Part model, mm, in its own coordinate system. A direction names the side the tool comes from. Give positions to 0.01 mm unless a question says otherwise; leave off trailing zeros. Order: outer loops, then holes, each group sorted by start corner. A loop starts at its lowest first (then second) coordinate and runs counter-clockwise, first axis right, second up. Notation, with made-up numbers: M 73.5,68 L 131.5,68 A19 ccw 131.5,75 Z; hole C 35,15.25 d2. An arc over 180 degrees is marked long. One line per question, with ' | ' between items.
```python
from build123d import *

# Parameters (mm, degrees)
SKETCH1_W               = 2200
SKETCH1_H               = 1000
BOSS_EXTRUDE1_DEPTH     = 1100
SKETCH2_W               = 2000
SKETCH2_H               = 900
CUT_EXTRUDE1_DEPTH      = 1
CUT_EXTRUDE1_DEPTH_BACK = 1101
FILLET1_R               = 50
CUT_EXTRUDE2_REACH      = 1002
SKETCH3_W               = 100
SKETCH3_H               = 900
SKETCH4_W               = 1000
SKETCH4_H               = 850
CUT_EXTRUDE3_DEPTH      = 1
CUT_EXTRUDE3_DEPTH_BACK = 2201


with BuildPart() as part:
    # Sketch1 → Boss-Extrude1 (new body)
    with BuildSketch(Plane.XY):
        with Locations((-1100, 500)):
            Rectangle(SKETCH1_W, SKETCH1_H)
    extrude(amount=BOSS_EXTRUDE1_DEPTH)

    # Sketch2 → Cut-Extrude1 (cut, two sides)
    with BuildSketch(Plane.XY.offset(1100)) as cut_extrude1_sk:
        with Locations((-1100, 500)):
            Rectangle(SKETCH2_W, SKETCH2_H)
    extrude(amount=CUT_EXTRUDE1_DEPTH, mode=Mode.SUBTRACT)
    extrude(cut_extrude1_sk.sketch, amount=-CUT_EXTRUDE1_DEPTH_BACK, mode=Mode.SUBTRACT)

    # Fillet1
    fillet1_edges = [part.edges().sort_by_distance(p)[0] for p in [
        (-2100, 50, 550),
        (-2100, 950, 550),
        (-100, 950, 550),
        (-100, 50, 550),
        (0, 0, 550),
        (-2200, 0, 550),
        (-2200, 1000, 550),
        (0, 1000, 550),
    ]]
    fillet(fillet1_edges, radius=FILLET1_R)

    # Sketch3 → Cut-Extrude2 (cut, up to next)
    with BuildSketch(Plane(origin=(0, 1000, 0), x_dir=(1, 0, 0), z_dir=(0, 1, 0)), mode=Mode.PRIVATE) as cut_extrude2_sk1:
        with Locations((-2000, -550)):
            Rectangle(SKETCH3_W, SKETCH3_H)
    cut_extrude2_tool1 = extrude(cut_extrude2_sk1.sketch, amount=-CUT_EXTRUDE2_REACH, mode=Mode.PRIVATE) & part.part
    add(cut_extrude2_tool1.solids().sort_by_distance((-2000, 1000, 550))[0], mode=Mode.SUBTRACT)
    # Sketch3 → Cut-Extrude2 (cut, up to next)
    with BuildSketch(Plane(origin=(0, 1000, 0), x_dir=(1, 0, 0), z_dir=(0, 1, 0)), mode=Mode.PRIVATE) as cut_extrude2_sk2:
        with Locations((-1800, -550)):
            Rectangle(SKETCH3_W, SKETCH3_H)
    cut_extrude2_tool2 = extrude(cut_extrude2_sk2.sketch, amount=-CUT_EXTRUDE2_REACH, mode=Mode.PRIVATE) & part.part
    add(cut_extrude2_tool2.solids().sort_by_distance((-1800, 1000, 550))[0], mode=Mode.SUBTRACT)
    # Sketch3 → Cut-Extrude2 (cut, up to next)
    with BuildSketch(Plane(origin=(0, 1000, 0), x_dir=(1, 0, 0), z_dir=(0, 1, 0)), mode=Mode.PRIVATE) as cut_extrude2_sk3:
        with Locations((-1600, -550)):
            Rectangle(SKETCH3_W, SKETCH3_H)
    cut_extrude2_tool3 = extrude(cut_extrude2_sk3.sketch, amount=-CUT_EXTRUDE2_REACH, mode=Mode.PRIVATE) & part.part
    add(cut_extrude2_tool3.solids().sort_by_distance((-1600, 1000, 550))[0], mode=Mode.SUBTRACT)
    # Sketch3 → Cut-Extrude2 (cut, up to next)
    with BuildSketch(Plane(origin=(0, 1000, 0), x_dir=(1, 0, 0), z_dir=(0, 1, 0)), mode=Mode.PRIVATE) as cut_extrude2_sk4:
        with Locations((-1400, -550)):
            Rectangle(SKETCH3_W, SKETCH3_H)
    cut_extrude2_tool4 = extrude(cut_extrude2_sk4.sketch, amount=-CUT_EXTRUDE2_REACH, mode=Mode.PRIVATE) & part.part
    add(cut_extrude2_tool4.solids().sort_by_distance((-1400, 1000, 550))[0], mode=Mode.SUBTRACT)
    # Sketch3 → Cut-Extrude2 (cut, up to next)
    with BuildSketch(Plane(origin=(0, 1000, 0), x_dir=(1, 0, 0), z_dir=(0, 1, 0)), mode=Mode.PRIVATE) as cut_extrude2_sk5:
        with Locations((-1200, -550)):
            Rectangle(SKETCH3_W, SKETCH3_H)
    cut_extrude2_tool5 = extrude(cut_extrude2_sk5.sketch, amount=-CUT_EXTRUDE2_REACH, mode=Mode.PRIVATE) & part.part
    add(cut_extrude2_tool5.solids().sort_by_distance((-1200, 1000, 550))[0], mode=Mode.SUBTRACT)
    # Sketch3 → Cut-Extrude2 (cut, up to next)
    with BuildSketch(Plane(origin=(0, 1000, 0), x_dir=(1, 0, 0), z_dir=(0, 1, 0)), mode=Mode.PRIVATE) as cut_extrude2_sk6:
        with Locations((-1000, -550)):
            Rectangle(SKETCH3_W, SKETCH3_H)
    cut_extrude2_tool6 = extrude(cut_extrude2_sk6.sketch, amount=-CUT_EXTRUDE2_REACH, mode=Mode.PRIVATE) & part.part
    add(cut_extrude2_tool6.solids().sort_by_distance((-1000, 1000, 550))[0], mode=Mode.SUBTRACT)
    # Sketch3 → Cut-Extrude2 (cut, up to next)
    with BuildSketch(Plane(origin=(0, 1000, 0), x_dir=(1, 0, 0), z_dir=(0, 1, 0)), mode=Mode.PRIVATE) as cut_extrude2_sk7:
        with Locations((-800, -550)):
            Rectangle(SKETCH3_W, SKETCH3_H)
    cut_extrude2_tool7 = extrude(cut_extrude2_sk7.sketch, amount=-CUT_EXTRUDE2_REACH, mode=Mode.PRIVATE) & part.part
    add(cut_extrude2_tool7.solids().sort_by_distance((-800, 1000, 550))[0], mode=Mode.SUBTRACT)
    # Sketch3 → Cut-Extrude2 (cut, up to next)
    with BuildSketch(Plane(origin=(0, 1000, 0), x_dir=(1, 0, 0), z_dir=(0, 1, 0)), mode=Mode.PRIVATE) as cut_extrude2_sk8:
        with Locations((-600, -550)):
            Rectangle(SKETCH3_W, SKETCH3_H)
    cut_extrude2_tool8 = extrude(cut_extrude2_sk8.sketch, amount=-CUT_EXTRUDE2_REACH, mode=Mode.PRIVATE) & part.part
    add(cut_extrude2_tool8.solids().sort_by_distance((-600, 1000, 550))[0], mode=Mode.SUBTRACT)
    # Sketch3 → Cut-Extrude2 (cut, up to next)
    with BuildSketch(Plane(origin=(0, 1000, 0), x_dir=(1, 0, 0), z_dir=(0, 1, 0)), mode=Mode.PRIVATE) as cut_extrude2_sk9:
        with Locations((-400, -550)):
            Rectangle(SKETCH3_W, SKETCH3_H)
    cut_extrude2_tool9 = extrude(cut_extrude2_sk9.sketch, amount=-CUT_EXTRUDE2_REACH, mode=Mode.PRIVATE) & part.part
    add(cut_extrude2_tool9.solids().sort_by_distance((-400, 1000, 550))[0], mode=Mode.SUBTRACT)
    # Sketch3 → Cut-Extrude2 (cut, up to next)
    with BuildSketch(Plane(origin=(0, 1000, 0), x_dir=(1, 0, 0), z_dir=(0, 1, 0)), mode=Mode.PRIVATE) as cut_extrude2_sk10:
        with Locations((-200, -550)):
            Rectangle(SKETCH3_W, SKETCH3_H)
    cut_extrude2_tool10 = extrude(cut_extrude2_sk10.sketch, amount=-CUT_EXTRUDE2_REACH, mode=Mode.PRIVATE) & part.part
    add(cut_extrude2_tool10.solids().sort_by_distance((-200, 1000, 550))[0], mode=Mode.SUBTRACT)

    # Sketch4 → Cut-Extrude3 (cut, two sides)
    with BuildSketch(Plane(origin=(0, 0, 0), x_dir=(0, 0, -1), z_dir=(1, 0, 0))) as cut_extrude3_sk:
        with Locations((-550, 500)):
            Rectangle(SKETCH4_W, SKETCH4_H)
    extrude(amount=CUT_EXTRUDE3_DEPTH, mode=Mode.SUBTRACT)
    extrude(cut_extrude3_sk.sketch, amount=-CUT_EXTRUDE3_DEPTH_BACK, mode=Mode.SUBTRACT)


solid = part.part
```
1. Mould opens along Z. For faces 1 (the flat face through (-2200, 65, 547)), 2 (the flat face through (-1105, 984, 1100)), 3 (the flat face through (-1950, 975, 556)) say: released by +Z, released by -Z, zero draft, split by the parting line, or undercut.
Worked out:
face 1: zero draft | face 2: released by +Z | face 3: undercut
2. Slice it at B-B on y = 560.5. Give the cut face in (x, z).
Worked out:
outline: M -2200,0 L -2100,0 L -2100,50 L -2200,50 Z; M -2200,1050 L -2100,1050 L -2100,1100 L -2200,1100 Z; M -100,0 L 0,0 L 0,50 L -100,50 Z; M -100,1050 L 0,1050 L 0,1100 L -100,1100 Z
3. Slice it at A-A on x = -1377. Give the cut face in (y, z).
Worked out:
outline: M 0,0 L 50,0 L 50,1100 L 0,1100 Z; M 950,0 L 1000,0 L 1000,100 L 950,100 Z; M 950,1000 L 1000,1000 L 1000,1100 L 950,1100 Z
4. Slice it at D-D on z = 947. Give the number of separate pieces and of enclosed holes in the cut face, then the cut area to 3 significant figures.
Worked out:
separate pieces: 12 | enclosed holes: 0 | area: 180,000 mm2
5. Drop flat-ended pins along their axis: pin 1 (1.5 mm diameter, centred on x = -1800, z = 498.5, fed in from +Y); pin 2 (15 mm diameter, centred on y = 975, z = 698, fed in from -X); pin 3 (25 mm diameter, centred on x = -604, y = 968, fed in from -Z); pin 4 (15 mm diameter, centred on y = 971.5, z = 438.5, fed in from +X). Give the stop position or say it passes through.
Worked out:
pin 1: stops at y = 50 | pin 2: stops at x = -2196.84 | pin 3: stops at z = 0 | pin 4: stops at x = -2
6. Slice it at C-C on x = -479. Give the cut face in (y, z).
Worked out:
outline: M 0,0 L 50,0 L 50,1100 L 0,1100 Z; M 950,0 L 1000,0 L 1000,1100 L 950,1100 Z
7. Tool access for faces 4 (the cylindrical face through (-15.036, 14.258, 557.7)), 5 (the flat face through (-2146, 75, 557)), 6 (the cylindrical face through (-2078.23, 941.27, 542.3)), 7 (the flat face through (-650, 975, 556)), 8 (the flat face through (0, 65, 547)): list every direction of +Z, -Z, +X, -X, +Y, -Y with a clear straight run to the whole face (end or side of a thin tool).
Worked out:
face 4: +Z, -Z, +X, -Y | face 5: +X, -X | face 6: +Z, -Z | face 7: +Y | face 8: +Z, -Z, +X, +Y, -Y
8. Probe L1, parallel to Y at x = -162.5, z = 61.5; L2, parallel to Z at x = -165, y = 955; L3, parallel to Y at x = -2065.5, z = 883.5. List the from-to ranges inside material, lowest first. Write a range as from..to.
Worked out:
L1: y = 0..50, 950..1000 | L2: z = 0..100, 1000..1100 | L3: y = 0..52.46, 947.54..1000
